from build123d import *

# Parameters (mm, degrees)
F0_R     = 7.8658205016
F0_R_2   = 8.0096944888
F1_DEPTH = 25.4
F2_W     = 54.2384404689
F2_H     = 12.1728531085
F3_DEPTH = 25.4
F5_DEPTH = 25.4
F6_R     = 3.3542510186
F7_DEPTH = 77.978


with BuildPart() as f1:
    # F0 (on Top) → F1 (new body)
    with BuildSketch(Plane.XY):
        with BuildLine():
            ThreePointArc((-47.5300452468, 0), (-54.0726039784, -12.3169262593), (-47.5300452468, -24.6338525186))
            Line((-47.5300452468, -24.6338525186), (58.5692822962, -24.6338525186))
            ThreePointArc((58.5692822962, -24.6338525186), (63.62716281, -12.3169262593), (58.5692822962, 0))
            Line((58.5692822962, 0), (-47.5300452468, 0))
        make_face()
        with Locations((-39.2074911675, -12.3169262593)):
            Circle(F0_R, mode=Mode.SUBTRACT)
        with Locations((46.10116281, -12.3169262593)):
            Circle(F0_R_2, mode=Mode.SUBTRACT)
    extrude(amount=F1_DEPTH)

    # F2 (on face) → F3 (join)
    with BuildSketch(Plane.XY.offset(25.4)):
        with Locations((2.7952184901, -12.50546542)):
            Rectangle(F2_W, F2_H)
    extrude(amount=F3_DEPTH)

    # F4 (on face) → F5 (cut)
    with BuildSketch(Plane(origin=(0, -6.4190388657, 0), x_dir=(-1, 0, 0), z_dir=(0, 1, 0))):
        with BuildLine():
            Line((15.5491959304, 50.8), (-20.8479575813, 50.8))
            Line((-20.8479575813, 50.8), (-20.8479575813, 33.394984901))
            ThreePointArc((-20.8479575813, 33.394984901), (-2.6493808255, 25.785842215), (15.5491959304, 33.394984901))
            Line((15.5491959304, 33.394984901), (15.5491959304, 50.8))
        make_face()
    extrude(amount=-F5_DEPTH, mode=Mode.SUBTRACT)

    # F6 (on face) → F7 (cut)
    with BuildSketch(Plane(origin=(-24.3240017444, 0, 0), x_dir=(0, -1, 0), z_dir=(-1, 0, 0))):
        with BuildLine():
            ThreePointArc((6.4190388657, 45.2219136059), (12.5051093125, 50.7371205343), (18.5918919742, 45.2226996422))
            Line((18.5918919742, 45.2226996422), (18.5918919742, 50.8))
            Line((18.5918919742, 50.8), (6.4190388657, 50.8))
            Line((6.4190388657, 50.8), (6.4190388657, 45.2219136059))
        make_face()
        with Locations((12.5055042435, 44.6210700417)):
            Circle(F6_R)
    extrude(amount=-F7_DEPTH, mode=Mode.SUBTRACT)


solid = f1.part
The model under review builds one solid part; all positions refer to its coordinate system, in mm. A direction names the side the tool comes from. Give positions to 0.01 mm unless a question says otherwise; leave off trailing zeros. Write each loop counter-clockwise with the first axis right and the second up, starting at its lowest first coordinate (ties: lowest second). Pieces come first, ordered by that corner, then holes.
1. Wall thickness on L1, parallel to X at y = -16.25, z = 46.5; L2, parallel to X at y = -19.5, z = 12; L3, parallel to X at y = -10.5, z = 19: over which ranges is each line inside the solid? List them lowest first.
2. Draft analysis for pull direction Y (two halves, no side actions). For faces 1 (the cylindrical face through (25.318, -12.379, 50.736)), 2 (the cylindrical face through (2.933, -12.42, 25.787)), 3 (the cylindrical face through (-19.998, -15.705, 45.629)), 4 (the flat face through (5, -24.634, 13)), state which applies: +Y half, -Y half, draft (parallel to the pull), parting line (faces both ways), or undercut.
3. Add section B-B, the plane y = -7.5. Write out the cut boundary in (x, z), plus the area to 3 significant figures.
4. Add section D-D, the plane x = -5. Write out the cut boundary in (y, z), plus the area to 3 significant figures.
5. Add section A-A, the plane z = 39. Write out the cut boundary in (x, y), plus the area to 3 significant figures.
6. Add section C-C, the plane x = 22. Write out the cut boundary in (y, z), plus the area to 3 significant figures.
7. Tool access review of faces 5 (the flat face through (29.914, -13, 35)), 6 (the flat face through (-4, -18.592, 26)), 7 (the flat face through (-4, -6.419, 26)), 8 (the flat face through (-24.324, -13, 35)), 9 (the flat face through (20.848, -12, 40)): name each direction out of +Z, -Z, +X, -X, +Y, -Y from which nothing blocks a thin tool from reaching the whole face with its end or side.
8. For P1, Ø9.5, axis at y = -14, z = 42.5, coming from the +X side; P2, Ø6, axis at y = -12.51, z = 44.62, coming from the +X side; P3, Ø5, axis at y = -19.5, z = 10, coming from the +X side; P4, Ø3.5, axis at y = -15.5, z = 39.5, coming from the -X side, all flat-tipped, find the tip position at first contact; note any pin that passes through.
Worked answers:
1. L1: x = -24.32 to -15.55, 20.85 to 29.91
1. L2: x = -52.22 to -42.41, -36 to 42.56, 49.64 to 62.09
1. L3: x = -53.96 to -46.86, -31.55 to 38.3, 53.9 to 63.53
2. face 1: parting line
2. face 2: draft
2. face 3: undercut
2. face 4: -Y half
3. outline: (-53.27, 0) - (-45.43, 0) - (-45.43, 25.4) - (-53.27, 25.4) - close; (-32.99, 0) - (39.7, 0) - (39.7, 25.4) - (29.91, 25.4) - (29.91, 48.14) - (20.85, 48.14) - (20.85, 33.39) arc R25.57 cw to (-15.55, 33.39) - (-15.55, 48.14) - (-24.32, 48.14) - (-24.32, 25.4) - (-32.99, 25.4) - close; (52.5, 0) - (62.95, 0) - (62.95, 25.4) - (52.5, 25.4) - close
3. area: 2,820 mm2
4. outline: (-24.63, 0) - (0, 0) - (0, 25.4) - (-6.42, 25.4) - (-6.42, 26.96) - (-18.59, 26.96) - (-18.59, 25.4) - (-24.63, 25.4) - close
4. area: 645 mm2
5. outline: (-24.32, -18.59) - (-15.55, -18.59) - (-15.55, -6.42) - (-24.32, -6.42) - close; (20.85, -18.59) - (29.91, -18.59) - (29.91, -6.42) - (20.85, -6.42) - close
5. area: 217 mm2
6. outline: (-24.63, 0) - (0, 0) - (0, 25.4) - (-6.42, 25.4) - (-6.42, 45.22) arc R6.12 ccw to (-18.59, 45.22) - (-18.59, 25.4) - (-24.63, 25.4) - close; hole circle Ø6.71 at (-12.51, 44.62)
6. area: 883 mm2
7. face 5: +Z, +X, +Y, -Y
7. face 6: +Z, +X, -X, -Y
7. face 7: +Z, +X, -X, +Y
7. face 8: +Z, -X, +Y, -Y
7. face 9: +Z, +Y, -Y
8. P1: stops at x = 29.91
8. P2: passes through
8. P3: stops at x = 62.99
8. P4: stops at x = -24.32
